Source: CAD feature listing. Evaluate the final solid. Frame: model axes, mm. Give positions to 0.01 mm unless a question says otherwise; leave off trailing zeros. Write each loop counter-clockwise with the first axis right and the second up, starting at its lowest first coordinate (ties: lowest second). Pieces come first, ordered by that corner, then holes. Notation, with made-up numbers: M 70,-23.5 L 122,-23.5 A14 cw 122,-15.5 Z; hole C 79,59 d3. An arc over 180 degrees is marked long. Return JSON: item names as keys, results as strings.
Autodesk Inventor part; units mm, degrees
ref_plane "작업 평면3" through (0, 2.2, 0) normal (0, -1, 0) x (1, 0, 0)
ref_plane "YZ Plane" through (0, 0, 0) normal (1, 0, 0) x (0, 1, 0)
ref_plane "XZ Plane" through (0, 0, 0) normal (0, 1, 0) x (-1, 0, 0)
sketch "스케치1" plane through (0, 0, 0) normal (0, 1, 0) x (-1, 0, 0)
  line L0 (-16.2959, 6.75) -> (-6.75, 16.2959)
  line L1 (-6.75, 16.2959) -> (6.75, 16.2959)
  line L2 (6.75, 16.2959) -> (16.2959, 6.75)
  line L3 (16.2959, 6.75) -> (16.2959, -6.75)
  line L4 (16.2959, -6.75) -> (6.75, -16.2959)
  line L5 (6.75, -16.2959) -> (-6.75, -16.2959)
  line L6 (-6.75, -16.2959) -> (-16.2959, -6.75)
  line L7 (-16.2959, -6.75) -> (-16.2959, 6.75)
  line L8 (19.4959, 8.0755) -> (19.4959, -8.0755)
  line L9 (19.4959, -8.0755) -> (8.0755, -19.4959)
  line L10 (8.0755, -19.4959) -> (-8.0755, -19.4959)
  line L11 (-8.0755, -19.4959) -> (-19.4959, -8.0755)
  line L12 (-19.4959, -8.0755) -> (-19.4959, 8.0755)
  line L13 (-19.4959, 8.0755) -> (-8.0755, 19.4959)
  line L14 (-8.0755, 19.4959) -> (8.0755, 19.4959)
  line L15 (8.0755, 19.4959) -> (19.4959, 8.0755)
  point P0 (0, 0)
  point P1 (0, 0)
  point P2 (0, 0)
  dimension "d0" = 13.5
  dimension "d1" = 3.2
extrude "돌출1" add sketch "스케치1" along normal blind 4.4 contours L0 L1 L2 L3 L4 L5 L6 L7 | L8 L9 L10 L11 L12 L13 L14 L15
sketch "스케치14" plane through (0, 4.4, 0) normal (0, 1, 0) x (1, 0, 0)
  line L0 (6.75, -16.2959) -> (-6.75, -16.2959)
  line L1 (-6.75, -16.2959) -> (-16.2959, -6.75)
  line L2 (-16.2959, -6.75) -> (-16.2959, 6.75)
  line L3 (-16.2959, 6.75) -> (-6.75, 16.2959)
  line L4 (-6.75, 16.2959) -> (6.75, 16.2959)
  line L5 (6.75, 16.2959) -> (16.2959, 6.75)
  line L6 (16.2959, 6.75) -> (16.2959, -6.75)
  line L7 (16.2959, -6.75) -> (6.75, -16.2959)
  line L8 (-7.5784, 18.2959) -> (7.5784, 18.2959)
  line L9 (7.5784, 18.2959) -> (18.2959, 7.5784)
  line L10 (18.2959, 7.5784) -> (18.2959, -7.5784)
  line L11 (18.2959, -7.5784) -> (7.5784, -18.2959)
  line L12 (7.5784, -18.2959) -> (-7.5784, -18.2959)
  line L13 (-7.5784, -18.2959) -> (-18.2959, -7.5784)
  line L14 (-18.2959, -7.5784) -> (-18.2959, 7.5784)
  line L15 (-18.2959, 7.5784) -> (-7.5784, 18.2959)
  line L16 (19.4959, -8.0755) -> (19.4959, 8.0755)
  point P0 (0, 0)
  point P1 (0, 0)
  point P2 (0, 0)
  dimension "d138" = 2
  dimension "d139" = 1.2
extrude "돌출16" cut sketch "스케치14" against normal blind 1.2
sketch "스케치15" plane through (0, 4.4, 0) normal (0, 1, 0) x (1, 0, 0)
  line L0 (-16.2959, -6.75) -> (-6.75, -16.2959)
  line L1 (-6.75, -16.2959) -> (6.75, -16.2959)
  line L2 (6.75, -16.2959) -> (16.2959, -6.75)
  line L3 (16.2959, -6.75) -> (16.2959, 6.75)
  line L4 (16.2959, 6.75) -> (6.75, 16.2959)
  line L5 (6.75, 16.2959) -> (-6.75, 16.2959)
  line L6 (-6.75, 16.2959) -> (-16.2959, 6.75)
  line L7 (-16.2959, 6.75) -> (-16.2959, -6.75)
  point P0 (0, 0)
extrude "돌출17" cut sketch "스케치15" against normal blind 0.6
sketch "스케치16" plane through (0, 3.8, 0) normal (0, 1, 0) x (1, 0, 0)
  line L0 (-6.2529, 15.0959) -> (6.2529, 15.0959)
  line L1 (6.2529, 15.0959) -> (15.0959, 6.2529)
  line L2 (15.0959, 6.2529) -> (15.0959, -6.2529)
  line L3 (15.0959, -6.2529) -> (6.2529, -15.0959)
  line L4 (6.2529, -15.0959) -> (-6.2529, -15.0959)
  line L5 (-6.2529, -15.0959) -> (-15.0959, -6.2529)
  line L6 (-15.0959, -6.2529) -> (-15.0959, 6.2529)
  line L7 (-15.0959, 6.2529) -> (-6.2529, 15.0959)
  line L8 (16.2959, 6.75) -> (16.2959, -6.75)
  point P0 (0, 0)
  point P1 (0, 0)
  dimension "d144" = 1.2
extrude "돌출18" cut sketch "스케치16" against normal up to surface (3.8 mm away)
fillet "모깎기2" radius 1.2 16 edges at (0, 4.4, -19.4959) (-13.7857, 4.4, -13.7857) (13.7857, 4.4, -13.7857) (19.4959, 4.4, 0) (13.7857, 4.4, 13.7857) (0, 4.4, 19.4959) (-13.7857, 4.4, 13.7857) (-19.4959, 4.4, 0) (-19.4959, 0, 0) (-13.7857, 0, 13.7857) (0, 0, 19.4959) (13.7857, 0, 13.7857) (-13.7857, 0, -13.7857) (0, 0, -19.4959) (19.4959, 0, 0) (13.7857, 0, -13.7857)
ref_plane "작업 평면3" through (0, 2.2, 0) normal (0, -1, 0) x (1, 0, 0)
mirror "미러6" about plane through (0, 2.2, 0) normal (0, -1, 0) of "돌출17", "돌출16"
properties part number "OV-PAM_ring_2"
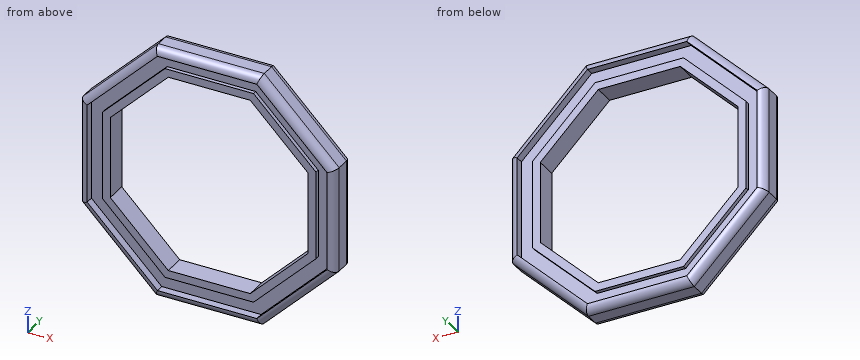
1) Line query: line 1 (Z direction, x = -1, y = 3.25); line 2 (Z direction, x = 0, y = 2.3). Output: solid intervals per line, ascending. Write a range as [from, to].
Numbers:
{"line 1": "z = [-19.49, -18.3], [-16.3, -15.1], [15.1, 16.3], [18.3, 19.49]", "line 2": "z = [-19.5, -15.1], [15.1, 19.5]"}
2) Contact query for flat-ended pins moving along their axis: pin 1 Ø10 at (x, z) = (13, -3) entering from -Y; pin 2 Ø0.6 at (x, y) = (1.5, 4) entering from +Z; pin 3 Ø1 at (x, y) = (-9.5, 3.5) entering from -Z. Output: stop coordinate, or through.
Numbers:
{"pin 1": "stops at y = 0.6", "pin 2": "stops at z = 19.39", "pin 3": "stops at z = -18.54"}
3) Cut plane C-C, the plane y = 2.3. Return the cut outline in (x, z).
Numbers:
{"outline": "M -19.5,-8.08 L -8.08,-19.5 L 8.08,-19.5 L 19.5,-8.08 L 19.5,8.08 L 8.08,19.5 L -8.08,19.5 L -19.5,8.08 Z; hole M -15.1,-6.25 L -6.25,-15.1 L 6.25,-15.1 L 15.1,-6.25 L 15.1,6.25 L 6.25,15.1 L -6.25,15.1 L -15.1,6.25 Z"}
